Design review of the part built by this model. Coordinates are the model's own, in mm. A direction names the side the tool comes from. Give positions to 0.01 mm unless a question says otherwise; leave off trailing zeros. Loops run counter-clockwise (first coordinate to the right, second up) from the corner with the lowest first, then second, coordinate; pieces in that order, holes last. Notation, with made-up numbers: M -11.5,32 L -5.5,32 A17 cw -5.5,58 Z; hole C -33,-6 d4. An arc over 180 degrees is marked long. Use a Markdown table: item, result. Add a question column.
(1) Insertion check: pin 1 Ø1.2 at (x, z) = (90.5, 2) entering from +Y; pin 2 Ø2 at (y, z) = (3, 3.5) entering from -X; pin 3 Ø11.5 at (x, y) = (22.5, 38.97) entering from -Z; pin 4 Ø1.2 at (x, z) = (29.5, 2.5) entering from +Y. Each pin has a flat end and moves straight along its axis. Give the tip position at first contact, or say it passes through.
(2) For probe 1 along Y at (x, z) = (59, 2.1) (3 decimals); probe 2 along Y at (x, z) = (22.5, 1.55); probe 3 along Y at (x, z) = (90, 1), list the stretches that pass through material, from the lowest coordinate up.
(3) Draft analysis for pull direction X (two halves, no side actions). For faces 4 (the face through (21.41, 34.06, 1.97)), 5 (the face through (14.31, 34.36, 1.97)), 6 (the face through (45.862, 22.087, 1.972)), 7 (the face through (31.87, 39.1, 1.97)), state which applies: pulls with the +X half, pulls with the -X half, needs draft (parallel to the pull), parting line crosses it, or undercut.
(4) Add section A-A, the plane y = 0. Give the boundary of the cut face in (x, z) (3 decimals), then the cut area to 3 significant figures.
(5) For faces 1 (the face through (64.015, 0, 2)), 2 (the face through (37, 3, 4)), 3 (the face through (92, 5.951, 2)), list the 3-axis set-ups (+Z, -Z, +X, -X, +Y, -Y) from which the entire face can be reached by the end or side of a thin tool; tool diameter is ignored.
(6) Add section B-B, the plane x = 90. Give the boundary of the cut face in (y, z).
(7) Add section C-C, the plane z = 0.8. State how many separate pieces and enclosed holes the cut face has, then the cut area to 3 significant figures.
(8) Add section D-D, the plane y = 15.5. Give the boundary of the cut face in (x, z), then the cut area to 3 significant figures.
```python
from build123d import *

# Parameters (mm, degrees)
SKETCH_1_R      = 5.03
SKETCH_1_R_2    = 1.5
SKETCH_1_W      = 8.03
SKETCH_1_H      = 4.03
EXTRUDE_1_DEPTH = 4


with BuildPart() as part:
    # 草图1 → 凸台-拉伸1 (new body)
    with BuildSketch(Plane.XY):
        with BuildLine():
            Line((87, -4.5), (9.367496998, -4.5))
            ThreePointArc((9.367496998, -4.5), (8.068458892, -4.795836543), (7.025622748, -5.625))
            ThreePointArc((7.025622748, -5.625), (-7.794228634, -4.5), (-1.358581522, 8.896867777))
            ThreePointArc((-1.358581522, 8.896867777), (-0.119086833, 9.385408641), (0.786634182, 10.36249037))
            Line((0.786634182, 10.36249037), (13.919137184, 33.108652801))
            ThreePointArc((13.919137184, 33.108652801), (14.312454275, 34.381571072), (14.11579573, 35.699275393))
            ThreePointArc((14.11579573, 35.699275393), (20.177098522, 47.666206639), (31.398879943, 40.316481698))
            ThreePointArc((31.398879943, 40.316481698), (31.879352208, 39.085435776), (32.842164256, 38.180272466))
            Line((32.842164256, 38.180272466), (87.068435314, 6.227425402))
            ThreePointArc((87.068435314, 6.227425402), (87.55756519, 6.02099445), (88.083774649, 5.950529007))
            Line((88.083774649, 5.950529007), (96, 5.950529007))
            ThreePointArc((96, 5.950529007), (97.414213562, 5.364742569), (98, 3.950529007))
            Line((98, 3.950529007), (98, 0))
            Line((98, 0), (98, -2.5))
            ThreePointArc((98, -2.5), (97.414213562, -3.914213562), (96, -4.5))
            Line((96, -4.5), (87, -4.5))
        make_face()
        Circle(SKETCH_1_R, mode=Mode.SUBTRACT)
        with Locations((22.5, 38.97114317)):
            Circle(SKETCH_1_R, mode=Mode.SUBTRACT)
        with Locations((30, 0)):
            Circle(SKETCH_1_R_2, mode=Mode.SUBTRACT)
        with Locations((90, 0)):
            Circle(SKETCH_1_R_2, mode=Mode.SUBTRACT)
        with Locations((60, 0)):
            Rectangle(SKETCH_1_W, SKETCH_1_H, mode=Mode.SUBTRACT)
        with BuildLine():
            Line((21.255373367, 27.815386605), (12.124355653, 12))
            ThreePointArc((12.124355653, 12), (12.124355653, 7), (16.454482672, 4.5))
            Line((16.454482672, 4.5), (58.367468971, 4.5))
            ThreePointArc((58.367468971, 4.5), (63.210197148, 8.25582003), (60.777559131, 13.880806481))
            Line((60.777559131, 13.880806481), (30.521886072, 30.525892321))
            ThreePointArc((30.521886072, 30.525892321), (28.338019103, 31.139965525), (26.107583087, 30.725820601))
            ThreePointArc((26.107583087, 30.725820601), (25.308251431, 30.420486827), (24.483535962, 30.192442521))
            ThreePointArc((24.483535962, 30.192442521), (22.620790776, 29.341612745), (21.255373367, 27.815386605))
        make_face(mode=Mode.SUBTRACT)
    extrude(amount=EXTRUDE_1_DEPTH)


solid = part.part
```
Established:
| question | item | result |
|---|---|---|
| 1 | pin 1 | y = 5.95 |
| 1 | pin 2 | x = -8.77 |
| 1 | pin 3 | z = 0 |
| 1 | pin 4 | y = 45.3 |
| 2 | probe 1 | -4.5 to -2.015, 2.015 to 4.54, 14.859 to 22.767 |
| 2 | probe 2 | -4.5 to 4.5, 29.25 to 33.94, 44 to 47.97 |
| 2 | probe 3 | -4.5 to -1.5, 1.5 to 5.95 |
| 3 | face 4 | undercut |
| 3 | face 5 | pulls with the -X half |
| 3 | face 6 | undercut |
| 3 | face 7 | pulls with the +X half |
| 4 | outline | M -9,0 L -5.03,0 L -5.03,4 L -9,4 Z; M 5.03,0 L 28.5,0 L 28.5,4 L 5.03,4 Z; M 31.5,0 L 55.985,0 L 55.985,4 L 31.5,4 Z; M 64.015,0 L 88.5,0 L 88.5,4 L 64.015,4 Z; M 91.5,0 L 98,0 L 98,4 L 91.5,4 Z |
| 4 | area | 332 mm^2 |
| 5 | face 1 | +Z, -Z |
| 5 | face 2 | +Z, +X, -X, +Y, -Y |
| 5 | face 3 | +Z, -Z, +X, +Y |
| 6 | outline | M -4.5,0 L -1.5,0 L -1.5,4 L -4.5,4 Z; M 1.5,0 L 5.95,0 L 5.95,4 L 1.5,4 Z |
| 7 | separate pieces | 1 |
| 7 | enclosed holes | 6 |
| 7 | area | 1,880 mm^2 |
| 8 | outline | M 3.75,0 L 14.15,0 L 14.15,4 L 3.75,4 Z; M 57.83,0 L 71.33,0 L 71.33,4 L 57.83,4 Z |
| 8 | area | 95.6 mm^2 |
